Drawing for the job (mm, zero at the part's lowest x, y, z). A direction names the side the tool comes from. Give positions to 0.01 mm unless a question says otherwise; leave off trailing zeros. Loops run counter-clockwise (first coordinate to the right, second up) from the corner with the lowest first, then second, coordinate; pieces in that order, holes last. Notation, with made-up numbers: (27.25, -32) -> (76.25, -32) arc R16 ccw to (76.25, -22) -> close; hole circle Ø3 at (37, -3). An arc over 180 degrees is marked (long way). Use CSV: the item, a comma, the result in double quotes. Start each with the question number.
(1) Cut at C-C on z = 5. Write the cut outline in (x, y), then the cut area to 3 significant figures.
(2) Pull direction Z, two halves, no side cores. Call the marked faces 1, 2, 3 and 4: pulls with the +Z half, pulls with the -Z half, needs draft (parallel to the pull), parting line crosses it, or undercut.
(3) Cut at A-A on x = 7.4. Write the cut outline in (y, z) (3 decimals), then the cut area to 3 significant figures.
(4) Drill centre lines: probe 1 along Z at (x, y) = (7.5, 1) (3 decimals); probe 2 along X at (y, z) = (3.35, 6.75); probe 3 along X at (y, z) = (5.3, 8.75). Where is each one in solid material? Low to high.
(5) 3-axis set-ups, long thin cutter, end or side, ignore diameter. For the marked faces 5, 6, 7, 8 and 9: which of +Z, -Z, +X, -X, +Y, -Y reach the whole face in a straight line?
(6) Flat gauge pins, fed straight in: pin 1 (3.5 mm diameter, centred on y = 3, z = 7, fed in from +X); pin 2 (2.5 mm diameter, centred on y = 3.5, z = 1, fed in from -X); pin 3 (1 mm diameter, centred on x = 13, y = 4.5, fed in from +Z). Where does each tip first touch, or does it go through?
(7) Cut at D-D on z = 12.75. Write the cut outline in (x, y).
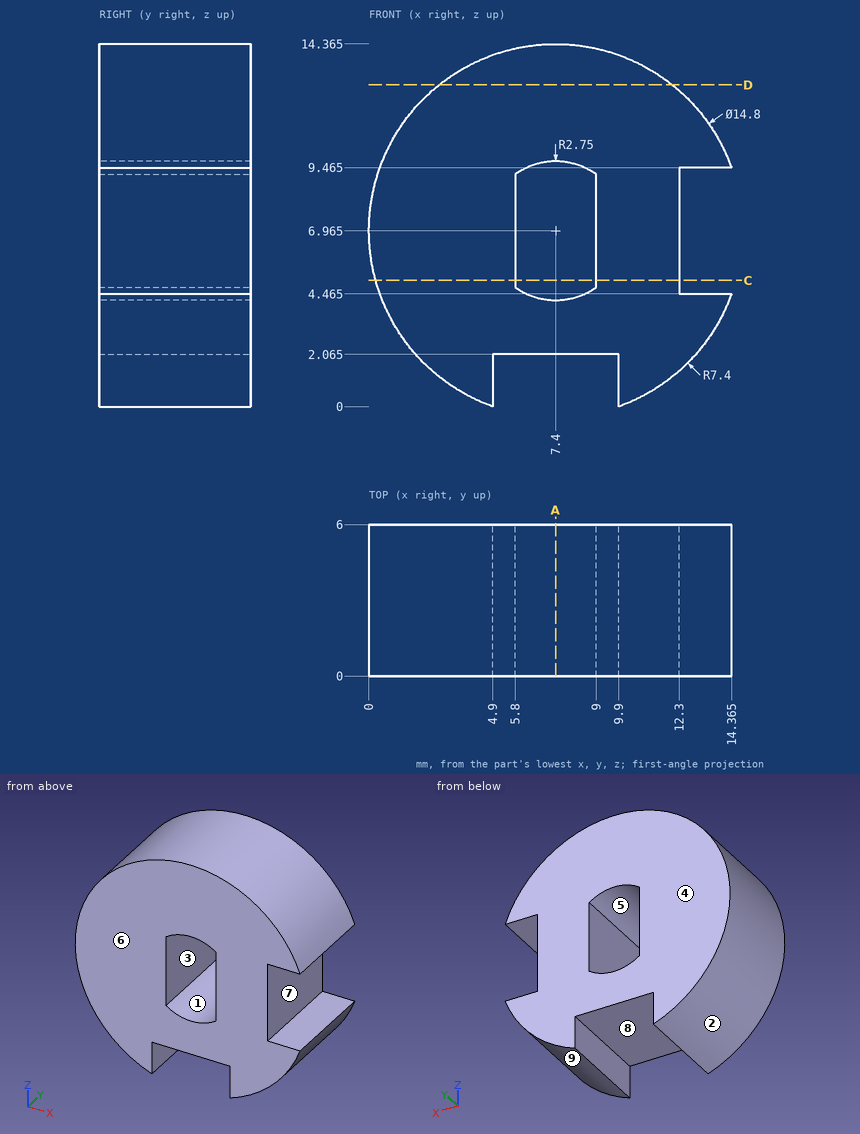
Check result:
1,outline,"(0.27, 0) -> (5.8, 0) -> (5.8, 6) -> (0.27, 6) -> close; (9, 0) -> (12.3, 0) -> (12.3, 6) -> (9, 6) -> close"
1,area,"53.0 mm²"
2,face 1,"undercut"
2,face 2,"parting line crosses it"
2,face 3,"undercut"
2,face 4,"needs draft"
3,outline,"(0, 2.065) -> (6, 2.065) -> (6, 4.215) -> (0, 4.215) -> close; (0, 9.715) -> (6, 9.715) -> (6, 14.365) -> (0, 14.365) -> close"
3,area,"40.8 mm²"
4,probe 1,"2.065 to 4.217, 9.713 to 14.364"
4,probe 2,"0 to 5.8, 9 to 12.3"
4,probe 3,"0.22 to 5.8, 9 to 12.3"
5,face 5,"+Y, -Y"
5,face 6,"+Z, -Z, +X, -X, -Y"
5,face 7,"+X, +Y, -Y"
5,face 8,"-Z, +Y, -Y"
5,face 9,"-Z, +X, +Y, -Y"
6,pin 1,"x = 12.3"
6,pin 2,"x = 1.7"
6,pin 3,"z = 12.33"
7,outline,"(2.79, 0) -> (12.01, 0) -> (12.01, 6) -> (2.79, 6) -> close"
